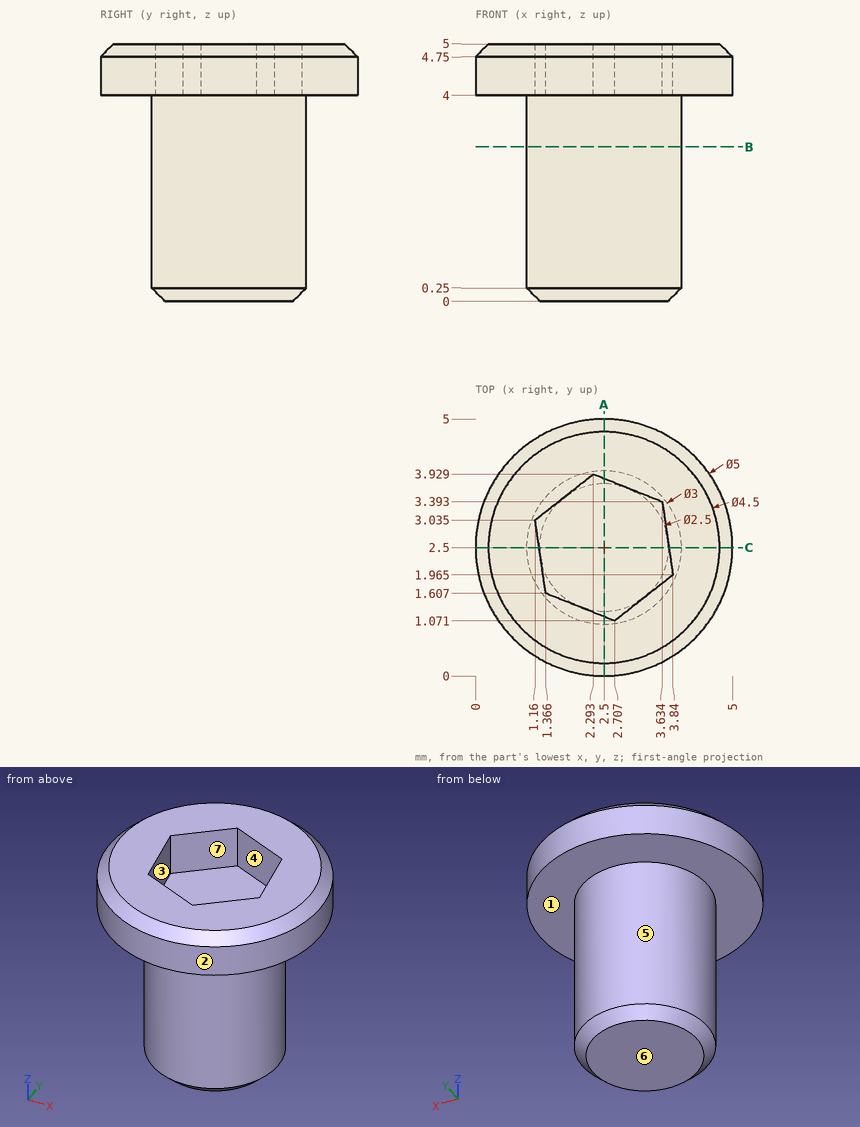
Drawing for the job (mm, zero at the part's lowest x, y, z). A direction names the side the tool comes from. Round coordinates to 2 decimals unless told otherwise and drop trailing zeros. Write each loop counter-clockwise with the first axis right and the second up, starting at its lowest first coordinate (ties: lowest second). Pieces come first, ordered by that corner, then holes. Notation, with made-up numbers: M 18.25,36.5 L 25.25,36.5 A36 ccw 25.25,74.5 Z; hole C -4,30 d6. An arc over 180 degrees is marked long. Put each result on its own line as item: value.
Item 1: Cut at C-C (y = 2.5). List the corners of the cut face in (x, z).
Responses:
outline: M 0,4 L 1,4 L 1,0.25 L 1.25,0 L 3.75,0 L 4,0.25 L 4,4 L 5,4 L 5,4.75 L 4.75,5 L 3.76,5 L 3.76,4 L 1.24,4 L 1.24,5 L 0.25,5 L 0,4.75 Z
Item 2: Cut at B-B (z = 3). List the corners of the cut face in (x, y).
Responses:
outline: C 2.5,2.5 d3
Item 3: Probe L1, parallel to Y at x = 2.55, z = 1.55; L2, parallel to Z at x = 2.2, y = 2.55. List the from-to ranges inside material, lowest first. Write a range as from..to.
Responses:
L1: 1..4
L2: 0..4
Item 4: Mould opens along X. For the marked faces 4, 5, 6 and 7 say: +X half, -X half, draft (parallel to the pull), parting line (faces both ways), or undercut.
Responses:
face 4: undercut
face 5: parting line
face 6: draft
face 7: undercut
Item 5: Cut at A-A (x = 2.5). List the corners of the cut face in (y, z).
Responses:
outline: M 0,4 L 1,4 L 1,0.25 L 1.25,0 L 3.75,0 L 4,0.25 L 4,4 L 5,4 L 5,4.75 L 4.75,5 L 3.85,5 L 3.85,4 L 1.15,4 L 1.15,5 L 0.25,5 L 0,4.75 Z
Item 6: Flat gauge pins, fed straight in: P1, Ø3, axis at x = 1.5, z = 1.5, coming from the +Y side; P2, Ø2, axis at x = 1, z = 4, coming from the -Y side; P3, Ø0.8, axis at x = 3, y = 3, coming from the +Z side. Where does each tip first touch, or does it go through?
Responses:
P1: y = 4
P2: y = 0.05
P3: z = 4
Item 7: Tool access for the marked faces 1, 2 and 3: list every direction of +Z, -Z, +X, -X, +Y, -Y with a clear straight run to the whole face (end or side of a thin tool).
Responses:
face 1: -Z
face 2: +Z, -Z
face 3: +Z
